Geometry: final body of the model. Coordinates: model frame, mm. Face numbers are marked on the shaded views. Give positions to 0.01 mm unless a question says otherwise; leave off trailing zeros. Order: outer loops, then holes, each group sorted by start corner. A loop starts at its lowest first (then second) coordinate and runs counter-clockwise, first axis right, second up. Notation, with made-up numbers: M -22.5,46 L -4.5,46 A25 cw -4.5,72 Z; hole C 47,87.5 d1. An arc over 180 degrees is marked long. One line per item, written item: value. Start each with the question number.
```python
from build123d import *

# Parameters (mm, degrees)
CUT_EXTRUDE1_DEPTH  = 9
SKETCH4_R           = 1.5
CUT_EXTRUDE10_DEPTH = 33.49


with BuildPart() as part:
    # Sketch2 → Revolve1 (revolve)
    with BuildSketch(Plane(origin=(0, 0, 0), x_dir=(0, 0, -1), z_dir=(1, 0, 0)), mode=Mode.PRIVATE) as revolve1_sk:
        with BuildLine():
            Line((-4.572036915, 0), (4.427963085, 0))
            Line((4.427963085, 0), (4.427963085, 35))
            Line((4.427963085, 35), (1.427963085, 35))
            Line((1.427963085, 35), (1.427963085, 33.49))
            ThreePointArc((1.427963085, 33.49), (-0.072036915, 31.99), (-1.572036915, 33.49))
            Line((-1.572036915, 33.49), (-1.572036915, 35))
            Line((-1.572036915, 35), (-4.572036915, 35))
            Line((-4.572036915, 35), (-4.572036915, 0))
        make_face()
    revolve(revolve1_sk.sketch.rotate(Axis((0, 0, 4.572036915), (0, 0, -1)), 90), axis=Axis((0, 0, 4.572036915), (0, 0, -1)))

    # Sketch3 → Cut-Extrude1 (cut)
    with BuildSketch(Plane(origin=(0, 0, -4.427963085), x_dir=(-1, 0, 0), z_dir=(0, 0, -1))):
        with BuildLine():
            Line((-2.613191437, 3.028403955), (2.678002471, 2.971245996))
            ThreePointArc((2.678002471, 2.971245996), (-0.043207356, -3.999766634), (-2.613191437, 3.028403955))
        make_face()
    extrude(amount=-CUT_EXTRUDE1_DEPTH, mode=Mode.SUBTRACT)

    # Sketch4 → Cut-Extrude10 (cut)
    with BuildSketch(Plane(origin=(0, 0, -4.427963085), x_dir=(-1, 0, 0), z_dir=(0, 0, -1))):
        with Locations((-5.81547747, 32.981211648)):
            Circle(SKETCH4_R)
        with Locations((5.81547747, 32.981211648)):
            Circle(SKETCH4_R)
    extrude(amount=-CUT_EXTRUDE10_DEPTH, mode=Mode.SUBTRACT)


solid = part.part
```
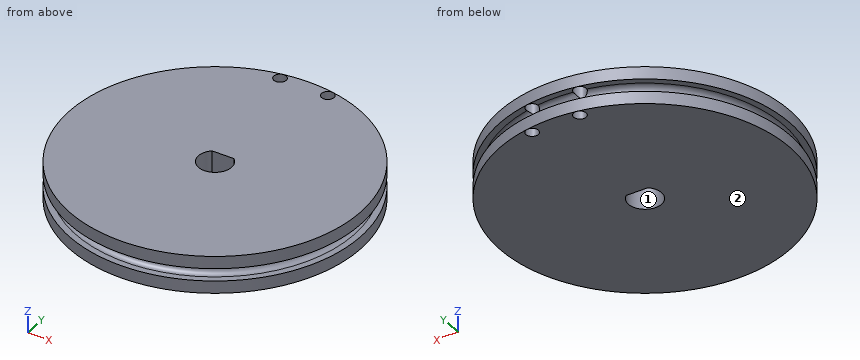
Q1. Ray query, line 1 along Z through (x, y) = (20.5, 27.5); line 2 along X through (y, z) = (0, 1.25); line 3 along Z through (x, y) = (-32, -8.5). Return the intervals inside material, ascending. Write a range as [from, to].
Q2. Section query B-B on x = 0. Return loops of the section in (y, z).
Q3. Section query C-C on z = -2.25. Return loops of the section in (x, y), and give its area (3 significant figures).
Q4. Contact query for flat-ended pins moving along their axis: pin 1 (5 mm diameter, centred on y = 16.5, z = 3, fed in from +X); pin 2 (1.5 mm diameter, centred on x = 26, z = 2.5, fed in from +Y); pin 3 (2.5 mm diameter, centred on x = 5.82, y = 32.98, fed in from -Z); pin 4 (1.5 mm diameter, centred on x = -16, z = -1.5, fed in from -Y). Output: stop coordinate, or through.
Q5. Section query A-A on y = 0. Return loops of the section in (x, z), and give its area (3 significant figures).
Q6. Mould query, pull axis Y, two halves, no side actions, for the marked faces 1 and 2. Classes: +Y half, -Y half, draft (parallel to the pull), parting line (faces both ways), or undercut.
Results below:
1. line 1: [-4.43, -1.43], [1.57, 4.57]
1. line 2: [-32.56, -4], [4, 32.56]
1. line 3: [-4.43, -1.38], [1.52, 4.57]
2. outline: M -35,-4.43 L -4,-4.43 L -4,4.57 L -35,4.57 L -35,1.57 L -33.49,1.57 A1.5 cw -33.49,-1.43 L -35,-1.43 Z; M 3,-4.43 L 35,-4.43 L 35,-1.43 L 33.49,-1.43 A1.5 cw 33.49,1.57 L 35,1.57 L 35,4.57 L 3,4.57 Z
3. outline: C 0,0 d70; hole C -5.82,32.98 d3; hole M -2.68,2.97 A4 ccw long 2.61,3.03 Z; hole C 5.82,32.98 d3
3. area: 3,790 mm2
4. pin 1: x = 32.08
4. pin 2: y = 24.24
4. pin 3: through
4. pin 4: y = -31.5
5. outline: M -35,-4.43 L -4,-4.43 L -4,4.57 L -35,4.57 L -35,1.57 L -33.49,1.57 A1.5 cw -33.49,-1.43 L -35,-1.43 Z; M 4,-4.43 L 35,-4.43 L 35,-1.43 L 33.49,-1.43 A1.5 cw 33.49,1.57 L 35,1.57 L 35,4.57 L 4,4.57 Z
5. area: 542 mm2
6. face 1: undercut
6. face 2: draft
